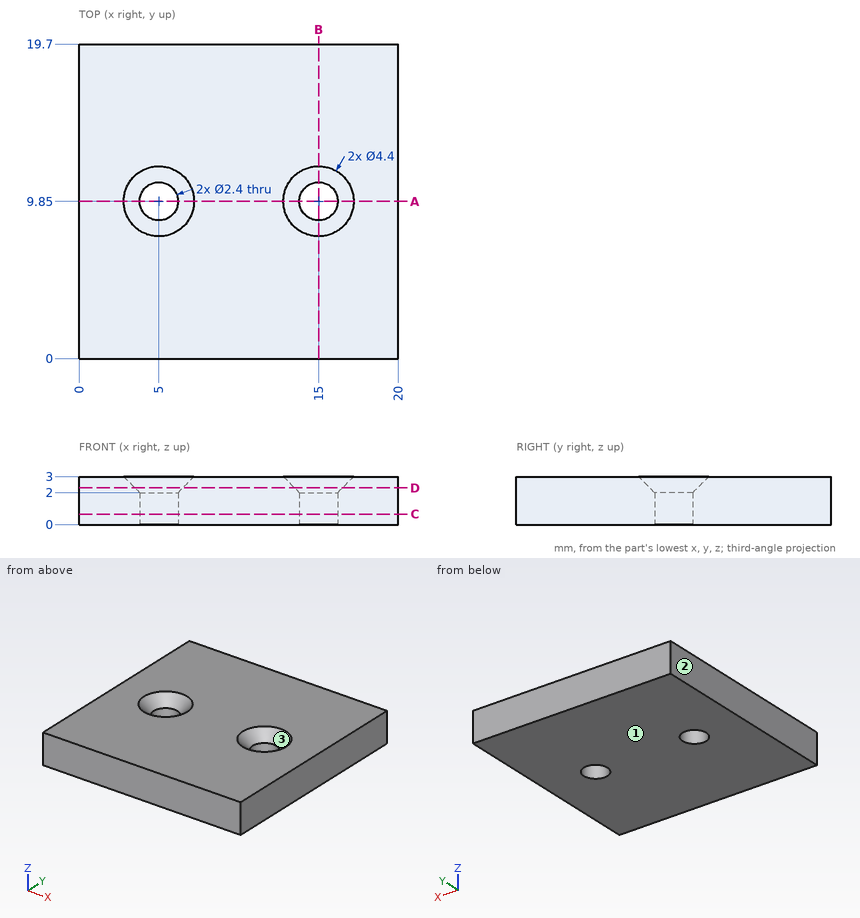
Answer from the drawing. Dimensions are ordinates in mm from the lowest x, y and z of the part. Coordinates: 2 decimals unless noted, no trailing zeros. Write each loop counter-clockwise with the first axis right and the second up, starting at its lowest first coordinate (ties: lowest second). Pieces come first, ordered by that corner, then holes. Notation, with made-up numbers: M -29,-28 L -20,-28 A26 ccw -20,-9 Z; hole C 87,15.25 d6. An arc over 180 degrees is marked long. Use one line per item in the form item = value. Start each with the question number.
1. The part is cut by section A-A (y = 9.85). Give the vertices of the cut face in (x, z), plus the area to 3 significant figures.
2. This flat-tipped pin is pushed along its axis until it touches: P1, Ø1.9, axis at x = 5, y = 9.85, coming from the -Z side. Where does it stop, or does it pass through?
3. The mould has two halves that part along X. Classify the marked faces 1, 2 and 3: released by +X, released by -X, zero draft, split by the parting line, or undercut.
4. The part is cut by section C-C (z = 0.65). Give the vertices of the cut face in (x, y), plus the area to 3 significant figures.
5. Straight lines are drawn through the part: probe 1 along X at (y, z) = (9.85, 0.85); probe 2 along Y at (x, z) = (15, 1.45); probe 3 along X at (y, z) = (9.75, 2.3). For each, find the intervals that lie inside material, in ascending order. Write a range as from..to.
6. The part is cut by section B-B (x = 15). Give the vertices of the cut face in (y, z), plus the area to 3 significant figures.
7. The part is cut by section D-D (z = 2.3). Give the vertices of the cut face in (x, y), plus the area to 3 significant figures.
Evaluation:
q1.outline = M 0,0 L 3.8,0 L 3.8,2 L 2.8,3 L 0,3 Z; M 6.2,0 L 13.8,0 L 13.8,2 L 12.8,3 L 7.2,3 L 6.2,2 Z; M 16.2,0 L 20,0 L 20,3 L 17.2,3 L 16.2,2 Z
q1.area = 43.6 mm^2
q2.P1 = through
q3.face_1 = zero draft
q3.face_2 = released by -X
q3.face_3 = undercut
q4.outline = M 0,0 L 20,0 L 20,19.7 L 0,19.7 Z; hole C 5,9.85 d2.4; hole C 15,9.85 d2.4
q4.area = 385 mm^2
q5.probe_1 = 0..3.8, 6.2..13.8, 16.2..20
q5.probe_2 = 0..8.65, 11.05..19.7
q5.probe_3 = 0..3.5, 6.5..13.5, 16.5..20
q6.outline = M 0,0 L 8.65,0 L 8.65,2 L 7.65,3 L 0,3 Z; M 11.05,0 L 19.7,0 L 19.7,3 L 12.05,3 L 11.05,2 Z
q6.area = 50.9 mm^2
q7.outline = M 0,0 L 20,0 L 20,19.7 L 0,19.7 Z; hole C 5,9.85 d3; hole C 15,9.85 d3
q7.area = 380 mm^2
